Source: three-view drawing plus pictorial views. Frame: mm from the lowest corner of the part. A direction names the side the tool comes from. Give positions to 0.01 mm unless a question says otherwise; leave off trailing zeros. Loops run counter-clockwise (first coordinate to the right, second up) from the corner with the lowest first, then second, coordinate; pieces in that order, holes last. Notation, with made-up numbers: M 61,-9 L 84,-9 A11 cw 84,12 Z; hole C 85.5,56 d4. An arc over 180 degrees is marked long. Write item = value, one per line.
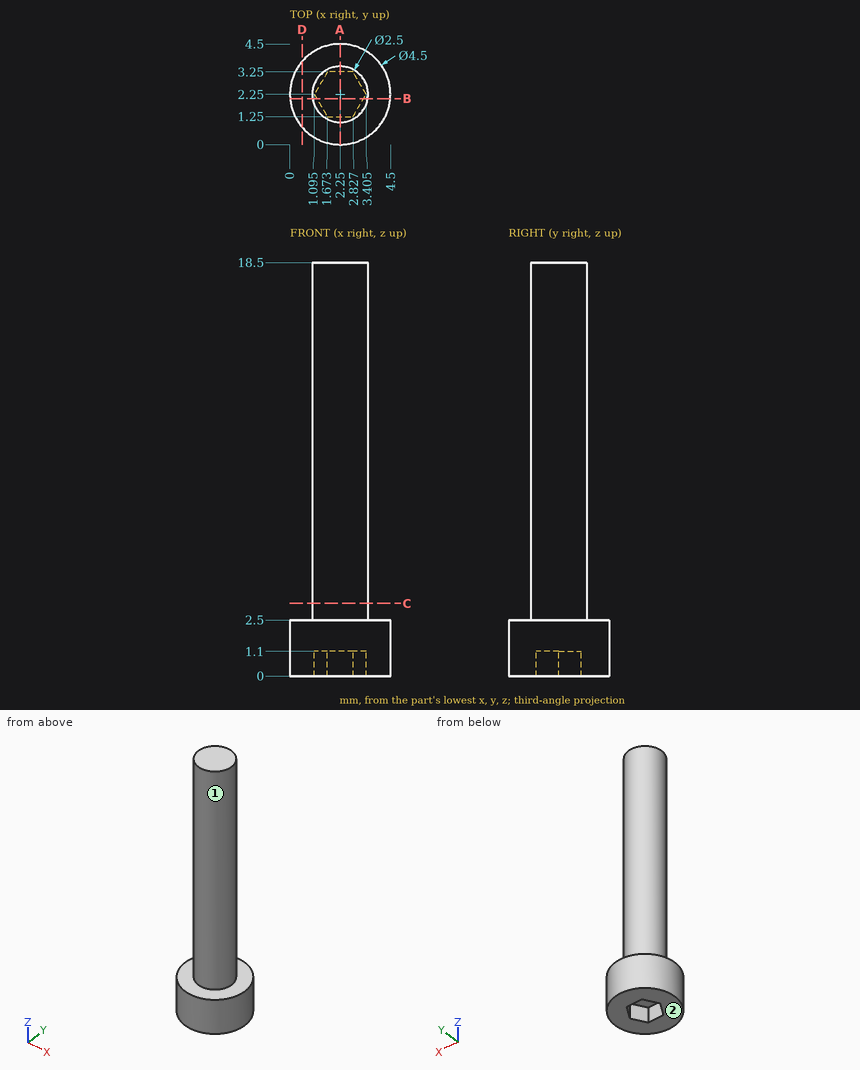
1. Cut plane D-D, the plane x = 0.55. Return the cut outline in (y, z).
Derived:
outline = M 0.78,0 L 3.72,0 L 3.72,2.5 L 0.78,2.5 Z
2. Material intervals for probe 1 along Z at (x, y) = (0.9, 3.1); probe 2 along Y at (x, z) = (2.2, 8.25); probe 3 along Z at (x, y) = (2.05, 1.85), sorted ascending. Write a range as from..to.
Derived:
probe_1 = 0..2.5
probe_2 = 1..3.5
probe_3 = 1.1..18.5
3. Cut plane C-C, the plane z = 3.25. Return the cut outline in (x, y).
Derived:
outline = C 2.25,2.25 d2.5
4. Reachability of the marked faces 1 and 2 from +Z, -Z, +X, -X, +Y, -Y: full face, straight path, thin tool, end or side. Return the list, or none.
Derived:
face_1 = +Z
face_2 = -Z, +X, -X, +Y, -Y
5. Cut plane B-B, the plane y = 2.05. Return the cut outline in (x, z).
Derived:
outline = M 0.01,0 L 1.21,0 L 1.21,1.1 L 3.29,1.1 L 3.29,0 L 4.49,0 L 4.49,2.5 L 3.48,2.5 L 3.48,18.5 L 1.02,18.5 L 1.02,2.5 L 0.01,2.5 Z
6. Cut plane A-A, the plane x = 2.25. Return the cut outline in (y, z).
Derived:
outline = M 0,0 L 1.25,0 L 1.25,1.1 L 3.25,1.1 L 3.25,0 L 4.5,0 L 4.5,2.5 L 3.5,2.5 L 3.5,18.5 L 1,18.5 L 1,2.5 L 0,2.5 Z
7. First-contact query: pin 1 Ø1 at (x, z) = (1.5, 16.5) entering from +Y (1 decimal); pin 2 Ø1.5 at (y, z) = (4, 3) entering from +X; pin 3 Ø1.5 at (y, z) = (4, 7.5) entering from -X. Flat tips, straight axial feed; report the tip coordinate or a pass-through.
Derived:
pin_1 = 3.5
pin_2 = 4.16
pin_3 = 1.5
